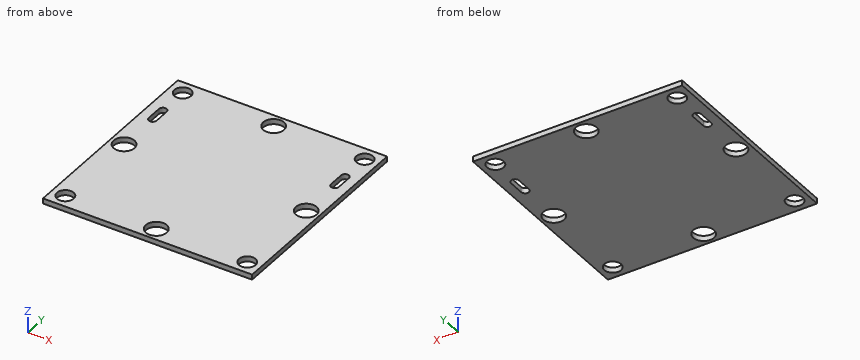
from build123d import *

# Parameters (mm, degrees)
SKETCH1_W           = 40
SKETCH1_H           = 40
BOSS_EXTRUDE1_DEPTH = 1
SKETCH2_R           = 1.6
SKETCH2_R_2         = 2
CUT_EXTRUDE1_DEPTH  = 10


with BuildPart() as part:
    # Sketch1 → Boss-Extrude1 (new body)
    with BuildSketch(Plane.XY):
        Rectangle(SKETCH1_W, SKETCH1_H)
    extrude(amount=BOSS_EXTRUDE1_DEPTH)

    # Sketch2 → Cut-Extrude1 (cut)
    with BuildSketch(Plane.XY.offset(1)):
        with Locations((-17.4, -17.4)):
            Circle(SKETCH2_R)
        with Locations((17.4, -17.4)):
            Circle(SKETCH2_R)
        with Locations((17.4, 17.4)):
            Circle(SKETCH2_R)
        with Locations((-17.4, 17.4)):
            Circle(SKETCH2_R)
        with Locations((0, 17.4)):
            Circle(SKETCH2_R_2)
        with Locations((17.450650527, 0)):
            Circle(SKETCH2_R_2)
        with Locations((0, -17.4)):
            Circle(SKETCH2_R_2)
        with Locations((-17.4, 0)):
            Circle(SKETCH2_R_2)
        with BuildLine():
            Line((-16.65, 11.5), (-16.65, 8.5))
            ThreePointArc((-16.65, 8.5), (-17.4, 7.75), (-18.15, 8.5))
            Line((-18.15, 8.5), (-18.15, 11.5))
            ThreePointArc((-18.15, 11.5), (-17.4, 12.25), (-16.65, 11.5))
        make_face()
        with BuildLine():
            Line((18.200650527, 11.5), (18.200650527, 8.5))
            ThreePointArc((18.200650527, 8.5), (17.450650527, 7.75), (16.700650527, 8.5))
            Line((16.700650527, 8.5), (16.700650527, 11.5))
            ThreePointArc((16.700650527, 11.5), (17.450650527, 12.25), (18.200650527, 11.5))
        make_face()
    extrude(amount=-CUT_EXTRUDE1_DEPTH, mode=Mode.SUBTRACT)


solid = part.part
The model under review builds one solid part; all positions refer to its coordinate system, in mm. Coordinates: 2 decimals unless noted, no trailing zeros. Write each loop counter-clockwise with the first axis right and the second up, starting at its lowest first coordinate (ties: lowest second). Pieces come first, ordered by that corner, then holes. Notation, with made-up numbers: (29.5, 83) - (39.5, 83) arc R18 ccw to (39.5, 109) - close; hole circle Ø6 at (68, -25.75). An arc over 180 degrees is marked (long way). Answer as CSV lines item,"result".
(1) We need section A-A (x = 0). Give the boundary of the cut face in (y, z).
Data:
outline,"(-20, 0) - (-19.4, 0) - (-19.4, 1) - (-20, 1) - close; (-15.4, 0) - (15.4, 0) - (15.4, 1) - (-15.4, 1) - close; (19.4, 0) - (20, 0) - (20, 1) - (19.4, 1) - close"
(2) For line 1 along Y through (x, z) = (17.4, 0.7); line 2 along Y through (x, z) = (-18, 0.85), list the stretches that pass through material, from the lowest coordinate up. Write a range as [from, to].
Data:
line 1,"y = [-20, -19], [-15.8, -2], [2, 7.75], [12.25, 15.8], [19, 20]"
line 2,"y = [-20, -18.88], [-15.92, -1.91], [1.91, 8.05], [11.95, 15.92], [18.88, 20]"
(3) We need section D-D (z = 0.35). Count the separate pieces of the cut face and the enclosed holes in it, plus the area to 3 significant figures.
Data:
separate pieces,"1"
enclosed holes,"10"
area,"1,510 mm2"
(4) We need section B-B (y = -17.4). Give the boundary of the cut face in (x, z), plus the area to 3 significant figures.
Data:
outline,"(-20, 0) - (-19, 0) - (-19, 1) - (-20, 1) - close; (-15.8, 0) - (-2, 0) - (-2, 1) - (-15.8, 1) - close; (2, 0) - (15.8, 0) - (15.8, 1) - (2, 1) - close; (19, 0) - (20, 0) - (20, 1) - (19, 1) - close"
area,"29.6 mm2"
(5) We need section C-C (y = 0). Give the boundary of the cut face in (x, z).
Data:
outline,"(-20, 0) - (-19.4, 0) - (-19.4, 1) - (-20, 1) - close; (-15.4, 0) - (15.45, 0) - (15.45, 1) - (-15.4, 1) - close; (19.45, 0) - (20, 0) - (20, 1) - (19.45, 1) - close"
